Here's how the part is built. I have some questions about the finished solid (model axes, mm). A direction names the side the tool comes from. Round coordinates to 2 decimals unless told otherwise and drop trailing zeros. Write each loop counter-clockwise with the first axis right and the second up, starting at its lowest first coordinate (ties: lowest second). Pieces come first, ordered by that corner, then holes. Notation, with made-up numbers: M -33.5,30.5 L 21.5,30.5 A24 cw 21.5,65.5 Z; hole C 42,-2.5 d2. An arc over 180 degrees is marked long. Use one line per item in the form item = value. Start each with the question number.
Q1. I want a section at C-C on y = 17.5. List the corners of the cut face in (x, z) for me, and give its area (3 significant figures).
Q2. I need wall thicknesses on line 1 along Y through (x, z) = (69.5, 6.25); line 2 along X through (y, z) = (-27.75, 7.75); line 3 along Y through (x, z) = (38, 7.75). Which ranges of each line are inside material? Lowest first, please. Write a range as from..to.
Q3. I want a section at D-D on x = -80.5. List the corners of the cut face in (y, z) for me, and give its area (3 significant figures).
Q4. We'd pull the mould along X, two halves only. Please class faces 1 (the face through (0, 31, 10)), 2 (the face through (71.5, 0, 6)), 3 (the face through (-1, -29.05, 6)): +X half, -X half, draft (parallel to the pull), parting line (faces both ways), or undercut.
Q5. For faces 4 (the face through (-1, 0, 1.8)), 5 (the face through (-1, -32.55, 6)), 6 (the face through (-1, 32.55, 6)), which set-ups out of +Z, -Z, +X, -X, +Y, -Y let a thin tool reach every point of the face, with its end or its side?
Q6. I'm going to push flat-ended pins straight in: pin 1 Ø4 at (x, z) = (21, 4.5) entering from +Y; pin 2 Ø2 at (x, y) = (-2, 2.5) entering from +Z; pin 3 Ø4 at (x, z) = (18, 4) entering from -Y. Where does each tip first touch, or does it pass through?
Q7. I want a section at B-B on x = -35.5. List the corners of the cut face in (y, z) for me.
Q8. I want a section at A-A on z = 7.5. List the corners of the cut face in (x, y) for me.
```python
from build123d import *

# Parameters (mm, degrees)
F0_W     = 185
F0_H     = 70
F0_W_2   = 143
F0_H_2   = 65.1
F0_R     = 1.25
F0_W_3   = 136
F0_H_3   = 58.1
F1_DEPTH = 1.8
F2_DEPTH = 10


with BuildPart() as f1:
    # F0 (on Top) → F1 (new body)
    with BuildSketch(Plane.XY):
        Rectangle(F0_W, F0_H)
        Rectangle(F0_W_2, F0_H_2, mode=Mode.SUBTRACT)
        Rectangle(F0_W_2, F0_H_2)
        with Locations((-69.5, -27.75)):
            Circle(F0_R, mode=Mode.SUBTRACT)
        with Locations((69.5, -27.75)):
            Circle(F0_R, mode=Mode.SUBTRACT)
        with Locations((-69.5, 29)):
            Circle(F0_R, mode=Mode.SUBTRACT)
        Rectangle(F0_W_3, F0_H_3, mode=Mode.SUBTRACT)
        with Locations((69.5, 29)):
            Circle(F0_R, mode=Mode.SUBTRACT)
        Rectangle(F0_W_3, F0_H_3)
        with Locations((-69.5, -27.75)):
            Circle(F0_R)
        with Locations((-69.5, 29)):
            Circle(F0_R)
        with Locations((69.5, 29)):
            Circle(F0_R)
        with Locations((69.5, -27.75)):
            Circle(F0_R)
    extrude(amount=F1_DEPTH)

    # F0 (on Top) → F2 (join)
    with BuildSketch(Plane.XY):
        Rectangle(F0_W_2, F0_H_2)
        with Locations((-69.5, -27.75)):
            Circle(F0_R, mode=Mode.SUBTRACT)
        with Locations((69.5, -27.75)):
            Circle(F0_R, mode=Mode.SUBTRACT)
        with Locations((-69.5, 29)):
            Circle(F0_R, mode=Mode.SUBTRACT)
        Rectangle(F0_W_3, F0_H_3, mode=Mode.SUBTRACT)
        with Locations((69.5, 29)):
            Circle(F0_R, mode=Mode.SUBTRACT)
    extrude(amount=F2_DEPTH)


solid = f1.part
```
Reported:
q1.outline = M -92.5,0 L 92.5,0 L 92.5,1.8 L 71.5,1.8 L 71.5,10 L 68,10 L 68,1.8 L -68,1.8 L -68,10 L -71.5,10 L -71.5,1.8 L -92.5,1.8 Z
q1.area = 390 mm^2
q2.line_1 = -32.55..-29, -26.5..27.75, 30.25..32.55
q2.line_2 = -71.5..-70.75, -68.25..-68, 68..68.25, 70.75..71.5
q2.line_3 = -32.55..-29.05, 29.05..32.55
q3.outline = M -35,0 L 35,0 L 35,1.8 L -35,1.8 Z
q3.area = 126 mm^2
q4.face_1 = draft
q4.face_2 = +X half
q4.face_3 = undercut
q5.face_4 = +Z
q5.face_5 = +Z, +X, -X, -Y
q5.face_6 = +Z, +X, -X, +Y
q6.pin_1 = 32.55
q6.pin_2 = 1.8
q6.pin_3 = -32.55
q7.outline = M -35,0 L 35,0 L 35,1.8 L 32.55,1.8 L 32.55,10 L 29.05,10 L 29.05,1.8 L -29.05,1.8 L -29.05,10 L -32.55,10 L -32.55,1.8 L -35,1.8 Z
q8.outline = M -71.5,-32.55 L 71.5,-32.55 L 71.5,32.55 L -71.5,32.55 Z; hole C -69.5,-27.75 d2.5; hole C -69.5,29 d2.5; hole M -68,-29.05 L 68,-29.05 L 68,29.05 L -68,29.05 Z; hole C 69.5,-27.75 d2.5; hole C 69.5,29 d2.5
